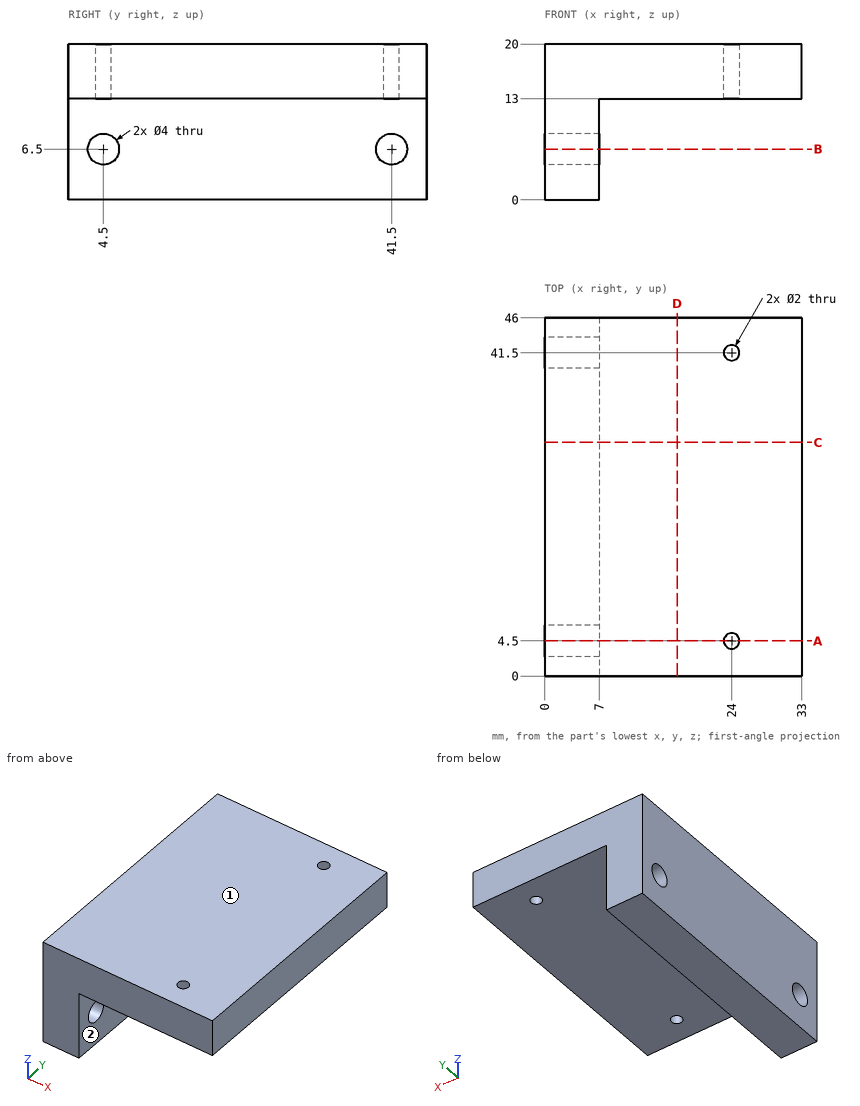
Source: three-view drawing plus pictorial views. Frame: mm from the lowest corner of the part. A direction names the side the tool comes from. Give positions to 0.01 mm unless a question says otherwise; leave off trailing zeros. Order: outer loops, then holes, each group sorted by start corner. A loop starts at its lowest first (then second) coordinate and runs counter-clockwise, first axis right, second up. Notation, with made-up numbers: M 46.5,5.5 L 103.5,5.5 A21 cw 103.5,36.5 Z; hole C 84,67.5 d2. An arc over 180 degrees is marked long. Return JSON: item names as keys, results as strings.
Item 1: Cut plane B-B (z = 6.5). Return loops of the section in (x, y), then the cut area to 3 significant figures.
Solutions:
{"outline": "M 0,0 L 7,0 L 7,2.5 L 0,2.5 Z; M 0,6.5 L 7,6.5 L 7,39.5 L 0,39.5 Z; M 0,43.5 L 7,43.5 L 7,46 L 0,46 Z", "area": "266 mm^2"}
Item 2: Cut plane D-D (x = 17). Return loops of the section in (y, z).
Solutions:
{"outline": "M 0,13 L 46,13 L 46,20 L 0,20 Z"}
Item 3: Cut plane C-C (y = 30). Return loops of the section in (x, z).
Solutions:
{"outline": "M 0,0 L 7,0 L 7,13 L 33,13 L 33,20 L 0,20 Z"}
Item 4: Access query for the marked faces 1 and 2. Directions: +Z, -Z, +X, -X, +Y, -Y. A direction counts if a zero-diameter tool reaches every point of the face in a straight line with its end or side. Return the directions, or none.
Solutions:
{"face 1": "+Z, +X, -X, +Y, -Y", "face 2": "-Z, +X, +Y, -Y"}
Item 5: First-contact query: P1, Ø4.5, axis at y = 41.5, z = 6.5, coming from the -X side; P2, Ø6.5, axis at y = 20, z = 9, coming from the +X side; P3, Ø6, axis at x = 16.5, y = 25.5, coming from the -Z side; P4, Ø5, axis at x = 10.5, z = 9, coming from the +Y side. Flat tips, straight axial feed; report the tip coordinate or a pass-through.
Solutions:
{"P1": "x = 0", "P2": "x = 7", "P3": "z = 13", "P4": "through"}
Item 6: Ray query, probe 1 along Y at (x, z) = (24, 14.75); probe 2 along Z at (x, y) = (3.75, 41.5); probe 3 along Z at (x, y) = (10.5, 22.5). Return the intervals inside material, ascending.
Solutions:
{"probe 1": "0 to 3.5, 5.5 to 40.5, 42.5 to 46", "probe 2": "0 to 4.5, 8.5 to 20", "probe 3": "13 to 20"}
Item 7: Cut plane A-A (y = 4.5). Return loops of the section in (x, z), then the cut area to 3 significant figures.
Solutions:
{"outline": "M 0,0 L 7,0 L 7,4.5 L 0,4.5 Z; M 0,8.5 L 7,8.5 L 7,13 L 23,13 L 23,20 L 0,20 Z; M 25,13 L 33,13 L 33,20 L 25,20 Z", "area": "280 mm^2"}
